```python
from build123d import *

# Parameters (mm, degrees)
SKETCH1_W                = 1300
SKETCH1_H                = 2400
BOSS_EXTRUDE1_DEPTH      = 60
CUT_EXTRUDE4_DEPTH       = 1100
CUT_EXTRUDE4_DEPTH_BACK  = 1100
BOSS_EXTRUDE2_DEPTH      = 100
BOSS_EXTRUDE2_DEPTH_BACK = 100
SKETCH7_W                = 55.5
SKETCH7_H                = 114
CUT_EXTRUDE5_DEPTH       = 3.4
CUT_EXTRUDE6_DEPTH       = 3.4
SKETCH13_W               = 195
SKETCH13_H               = 40
CUT_EXTRUDE7_DEPTH       = 5


with BuildPart() as part:
    # Sketch1 → Boss-Extrude1 (new body)
    with BuildSketch(Plane.XY):
        with Locations((90.331491713, 213.812154696)):
            Rectangle(SKETCH1_W, SKETCH1_H)
    extrude(amount=BOSS_EXTRUDE1_DEPTH)

    # Sketch5 → Cut-Extrude4 (cut, two sides)
    with BuildSketch(Plane(origin=(0, 213.812154696, 0), x_dir=(-1, 0, 0), z_dir=(0, -1, 0))) as cut_extrude4_sk:
        Polygon((-190.331491713, 0), (-235.364812709, -26), (-595.298170716, -26), (-640.331491713, 0), align=None)
        Polygon((9.668508287, 0), (459.668508287, 0), (414.635187291, -26), (54.701829284, -26), align=None)
        Polygon((414.635187291, -34), (459.668508287, -60), (9.668508287, -60), (54.701829284, -34), align=None)
        Polygon((-190.331491713, -60), (-235.364812709, -34), (-595.298170716, -34), (-640.331491713, -60), align=None)
    extrude(amount=CUT_EXTRUDE4_DEPTH, mode=Mode.SUBTRACT)
    extrude(cut_extrude4_sk.sketch, amount=-CUT_EXTRUDE4_DEPTH_BACK, mode=Mode.SUBTRACT)

    # Sketch6 → Boss-Extrude2 (add, two sides)
    with BuildSketch(Plane(origin=(0, 213.812154696, 0), x_dir=(-1, 0, 0), z_dir=(0, -1, 0))) as boss_extrude2_sk:
        Polygon((-190.331491713, 0), (-235.364812709, -26), (-595.298170716, -26), (-640.331491713, 0), align=None)
        Polygon((9.668508287, 0), (459.668508287, 0), (414.635187291, -26), (54.701829284, -26), align=None)
        Polygon((414.635187291, -34), (459.668508287, -60), (9.668508287, -60), (54.701829284, -34), align=None)
        Polygon((-190.331491713, -60), (-235.364812709, -34), (-595.298170716, -34), (-640.331491713, -60), align=None)
    extrude(amount=BOSS_EXTRUDE2_DEPTH)
    extrude(boss_extrude2_sk.sketch, amount=-BOSS_EXTRUDE2_DEPTH_BACK)

    # Sketch7 → Cut-Extrude5 (cut)
    with BuildSketch(Plane(origin=(0, 0, 0), x_dir=(-1, 0, 0), z_dir=(0, 0, -1))):
        with Locations((-712.581491713, 1256.812154696)):
            Rectangle(SKETCH7_W, SKETCH7_H)
        with Locations((-712.581491713, -829.187845304)):
            Rectangle(SKETCH7_W, SKETCH7_H)
        Polygon((474.668508287, 313.812154696), (529.668508287, 313.812154696), (539.668508287, 303.812154696), (539.668508287, 53.812154696), (529.668508287, 43.812154696), (474.668508287, 43.812154696), (464.668508287, 53.812154696), (464.668508287, 303.812154696), align=None)
    extrude(amount=-CUT_EXTRUDE5_DEPTH, mode=Mode.SUBTRACT)

    # Sketch10 → Cut-Extrude6 (cut)
    with BuildSketch(Plane.XY.offset(60)):
        Polygon((-529.668508287, 313.812154696), (-474.668508287, 313.812154696), (-464.668508287, 303.812154696), (-464.668508287, 53.812154696), (-474.668508287, 43.812154696), (-529.668508287, 43.812154696), (-539.668508287, 53.812154696), (-539.668508287, 303.812154696), align=None)
    extrude(amount=-CUT_EXTRUDE6_DEPTH, mode=Mode.SUBTRACT)

    # Sketch13 → Cut-Extrude7 (cut)
    with BuildSketch(Plane(origin=(0, 0, 0), x_dir=(-1, 0, 0), z_dir=(0, 0, -1))):
        with Locations((-499.186786697, -952.846120584)):
            Rectangle(SKETCH13_W, SKETCH13_H)
    extrude(amount=-CUT_EXTRUDE7_DEPTH, mode=Mode.SUBTRACT)


solid = part.part
```
The listing builds one solid part. Answer for the finished solid, in the listing's coordinates (mm). A direction names the side the tool comes from. Coordinates: 2 decimals unless noted, no trailing zeros. Write each loop counter-clockwise with the first axis right and the second up, starting at its lowest first coordinate (ties: lowest second). Pieces come first, ordered by that corner, then holes. Notation, with made-up numbers: (60, -16) - (92, -16) arc R14 ccw to (92, 2) - close; hole circle Ø9 at (-2, 71.5). An arc over 180 degrees is marked (long way). Return JSON: item names as keys, results as strings. Group by question number.
1. Which of the six approach directions +Z, -Z, +X, -X, +Y, -Y give full straight-line access (tool end or side, diameter ignored) to faces 1 (the flat face through (413, -379, 26)), 2 (the flat face through (212.5, 820.8, 47.2)), 3 (the flat face through (713, -828, 3.4))?
2. A cutting plane is placed at B-B, the plane x = -392.5. Determine the outline of the cut face in (y, z).
3. A cutting plane is placed at C-C, the plane z = 16. Determine the outline of the cut face in (x, y).
4. A cutting plane is placed at D-D, the plane x = 558.5. Determine the outline of the cut face in (y, z), plus the area to 3 significant figures.
5. Straight lines are drawn through the part: L1, parallel to Y at x = -223, z = 15; L2, parallel to Y at x = 582, z = 3; L3, parallel to X at y = 727, z = 21. For each, find the intervals that lie inside material, in ascending order.
6. Determine the mould class of faces 4 (the flat face through (-559.669, 197, 30)), 5 (the flat face through (-237, 807, 26)) for opening direction Y: released by +Y, released by -Y, zero draft, split by the parting line, or undercut.
7. Given pin 1 (3 mm diameter, centred on x = 222.5, y = 1139, fed in from +Z); pin 2 (12 mm diameter, centred on x = 462.5, y = -947.5, fed in from -Z); pin 3 (3.5 mm diameter, centred on y = 1237.5, z = 1.5, fed in from +X), each flat-ended and moving along its own axis, determine where each tip first touches the part or whether it passes through.
8. A cutting plane is placed at A-A, the plane y = -64.5. Determine the outline of the cut face in (x, z).
Ans:
{
 "1": {"face 1": "-Z", "face 2": "+Z", "face 3": "-Z, +X"},
 "2": {"outline": "(-986.19, 0) - (-886.19, 0) - (-886.19, 26) - (113.81, 26) - (113.81, 0) - (313.81, 0) - (313.81, 26) - (1313.81, 26) - (1313.81, 0) - (1413.81, 0) - (1413.81, 60) - (1313.81, 60) - (1313.81, 34) - (313.81, 34) - (313.81, 60) - (113.81, 60) - (113.81, 34) - (-886.19, 34) - (-886.19, 60) - (-986.19, 60) - close"},
 "3": {"outline": "(-559.67, -986.19) - (740.33, -986.19) - (740.33, 1413.81) - (-559.67, 1413.81) - close; hole (-431.96, -886.19) - (-37.38, -886.19) - (-37.38, 113.81) - (-431.96, 113.81) - close; hole (-431.96, 313.81) - (-37.38, 313.81) - (-37.38, 1313.81) - (-431.96, 1313.81) - close; hole (218.04, -886.19) - (612.62, -886.19) - (612.62, 113.81) - (218.04, 113.81) - close; hole (218.04, 313.81) - (612.62, 313.81) - (612.62, 1313.81) - (218.04, 1313.81) - close"},
 "4": {"outline": "(-986.19, 0) - (-972.85, 0) - (-972.85, 5) - (-932.85, 5) - (-932.85, 0) - (-886.19, 0) - (-886.19, 26) - (113.81, 26) - (113.81, 0) - (313.81, 0) - (313.81, 26) - (1313.81, 26) - (1313.81, 0) - (1413.81, 0) - (1413.81, 60) - (1313.81, 60) - (1313.81, 34) - (313.81, 34) - (313.81, 60) - (113.81, 60) - (113.81, 34) - (-886.19, 34) - (-886.19, 60) - (-986.19, 60) - close", "area": "39,800 mm²"},
 "5": {"L1": "-986.19 to -886.19, 113.81 to 313.81, 1313.81 to 1413.81", "L2": "-986.19 to -972.85, -932.85 to -886.19, 113.81 to 313.81, 1313.81 to 1413.81", "L3": "-559.67 to -423.3, -46.04 to 226.7, 603.96 to 740.33"},
 "6": {"face 4": "zero draft", "face 5": "undercut"},
 "7": {"pin 1": "z = 42.29", "pin 2": "z = 5", "pin 3": "x = 684.83"},
 "8": {"outline": "(-559.67, 0) - (-459.67, 0) - (-414.64, 26) - (-54.7, 26) - (-9.67, 0) - (190.33, 0) - (235.36, 26) - (595.3, 26) - (640.33, 0) - (740.33, 0) - (740.33, 60) - (640.33, 60) - (595.3, 34) - (235.36, 34) - (190.33, 60) - (-9.67, 60) - (-54.7, 34) - (-414.64, 34) - (-459.67, 60) - (-559.67, 60) - close"}
}
